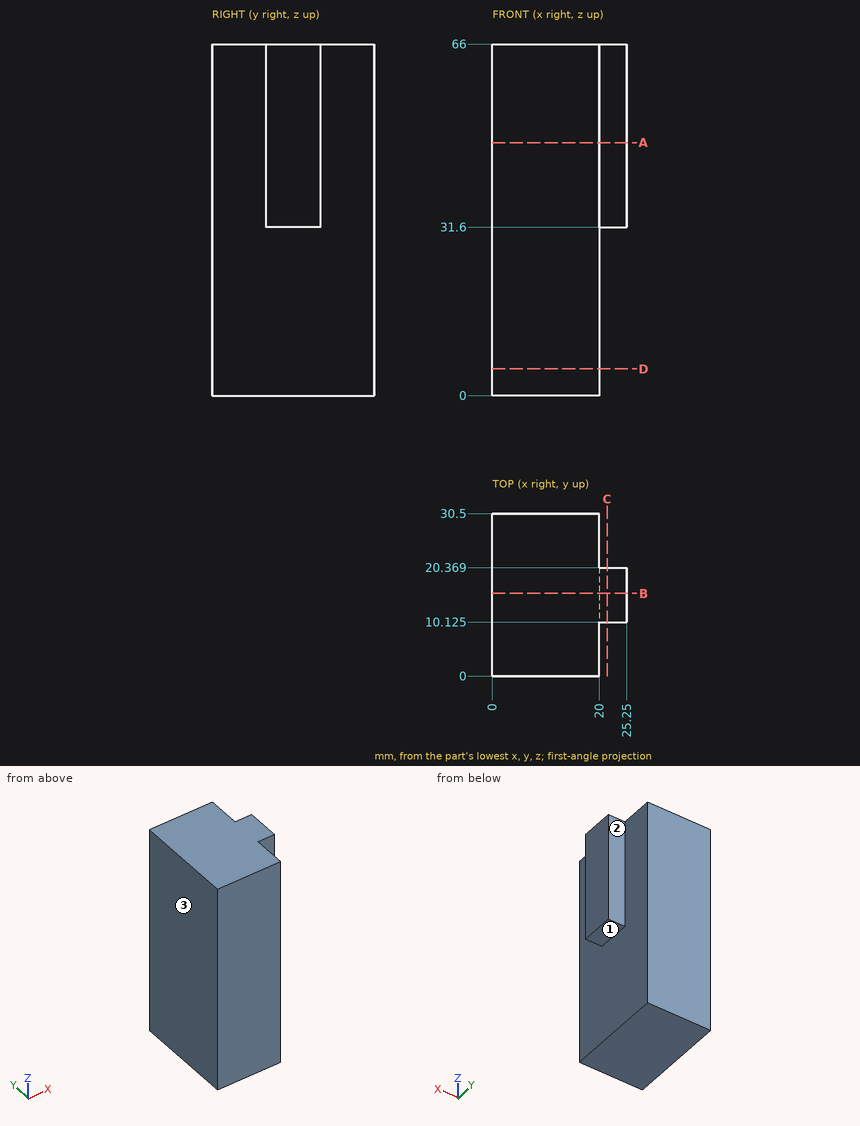
Study the drawing (mm; zero at the part's minimum x, y, z) and answer. A direction names the side the tool comes from. Give positions to 0.01 mm unless a question says otherwise; leave off trailing zeros. Write each loop counter-clockwise with the first axis right and the second up, starting at its lowest first coordinate (ties: lowest second). Pieces come first, ordered by that corner, then holes. Notation, with made-up numbers: (-17.75, 20) - (25.25, 20) arc R24 ccw to (25.25, 53) - close; hole circle Ø8 at (39.5, -4.75). An arc over 180 degrees is marked (long way). One line per question, with ' | ' between items. Start each with the question number.
1. For the marked faces 1, 2 and 3, determine the directions among +Z, -Z, +X, -X, +Y, -Y from which every point of the face is accessible in a straight line to the end or side of a thin tool.
2. Straight lines are drawn through the part: line 1 (Z direction, x = 22, y = 19); line 2 (X direction, y = 23.5, z = 28); line 3 (Y direction, x = 23.75, z = 50) (3 decimals). For each, find the intervals that lie inside material, in ascending order.
3. Section C-C, the plane x = 21.5 is taken. Determine the outline of the cut face in (y, z) (3 decimals).
4. Given P1, Ø4, axis at x = 23.5, z = 51.5, coming from the +Y side; P2, Ø2.5, axis at x = 22, z = 49, coming from the -Y side (3 decimals); P3, Ø10, axis at y = 5, z = 28, coming from the +X side, each flat-ended and moving along its own axis, determine where each tip first touches the part or whether it passes through.
5. Section B-B, the plane y = 15.5 is taken. Determine the outline of the cut face in (x, z), then the cut area to 3 significant figures.
6. Section A-A, the plane z = 47.5 is taken. Determine the outline of the cut face in (x, y) (3 decimals).
7. Section D-D, the plane z = 5 is taken. Determine the outline of the cut face in (x, y), then the cut area to 3 significant figures.
Result:
1) face 1: -Z, +X, +Y, -Y | face 2: +Z, -Z, +X, +Y | face 3: +Z, -Z, -X, +Y, -Y
2) line 1: z = 31.6 to 66 | line 2: x = 0 to 20 | line 3: y = 10.125 to 20.369
3) outline: (10.125, 31.6) - (20.369, 31.6) - (20.369, 66) - (10.125, 66) - close
4) P1: stops at y = 20.37 | P2: stops at y = 10.125 | P3: stops at x = 20
5) outline: (0, 0) - (20, 0) - (20, 31.6) - (25.25, 31.6) - (25.25, 66) - (0, 66) - close | area: 1,500 mm2
6) outline: (0, 0) - (20, 0) - (20, 10.125) - (25.25, 10.125) - (25.25, 20.369) - (20, 20.369) - (20, 30.5) - (0, 30.5) - close
7) outline: (0, 0) - (20, 0) - (20, 30.5) - (0, 30.5) - close | area: 610 mm2
